Could you check a few things on this drawing? It's one solid part, dimensions in mm from its lowest x, y, z. A direction names the side the tool comes from. Give positions to 0.01 mm unless a question says otherwise; leave off trailing zeros. Order: outer loops, then holes, each group sorted by start corner. A loop starts at its lowest first (then second) coordinate and runs counter-clockwise, first axis right, second up. Notation, with made-up numbers: M 73,24.25 L 115,24.25 A13 cw 115,30.25 Z; hole C 30,53 d9. An arc over 180 degrees is marked long. Return JSON: item names as keys, results as strings. Group by question number.
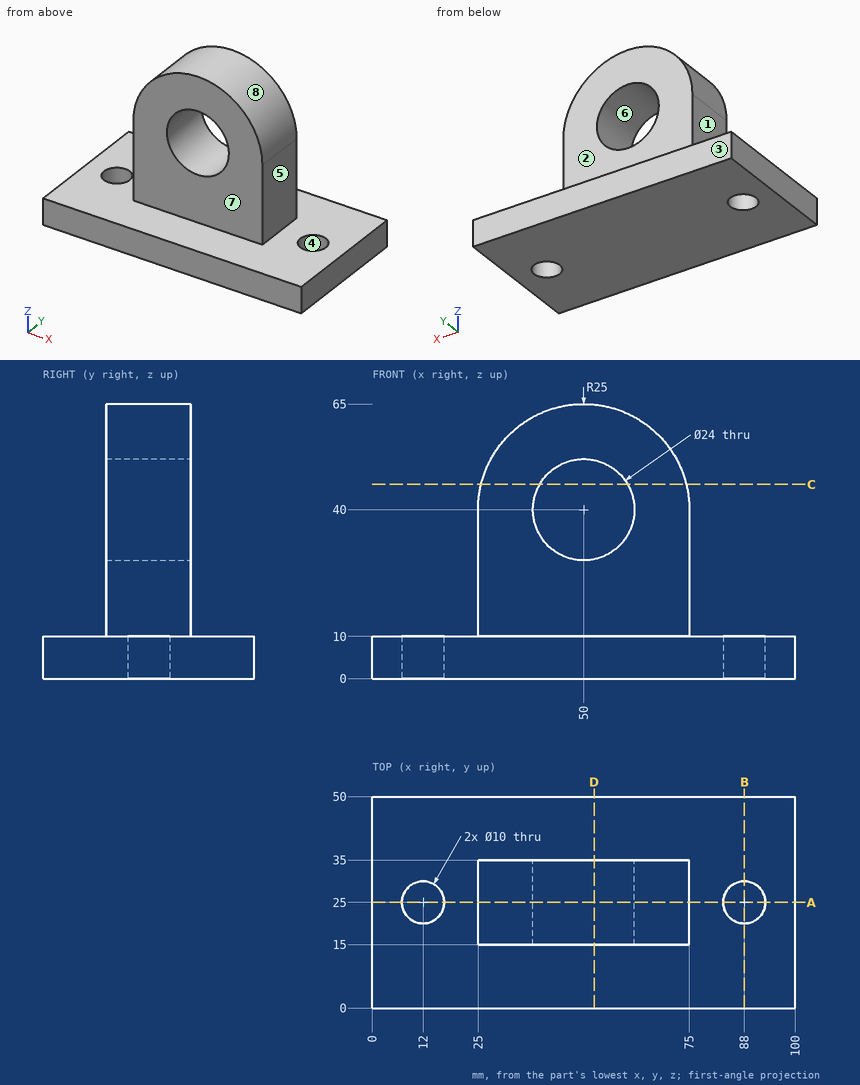
1. Imagine slicing it at A-A, the plane y = 25. Please give me the cut outline in (x, z), plus the area to 3 significant figures.
2. Imagine slicing it at D-D, the plane x = 52.5. Please give me the cut outline in (y, z).
3. Which directions (+Z, -Z, +X, -X, +Y, -Y) give clear straight access to the entire face, cutting with the end or side of a thin tool? Please do the marked faces 1, 2, 3, 4 and 5.
4. Imagine slicing it at C-C, the plane z = 46. Please give me the cut outline in (x, y).
5. I need wall thicknesses on L1, parallel to X at y = 25, z = 7.5; L2, parallel to X at y = 27, z = 40; L3, parallel to Y at x = 12, z = 2.75. Which ranges of each line are inside material? Lowest first, please. Write a range as from..to.
6. For pin 1 (6 mm diameter, centred on x = 38.5, y = 37.5, fed in from -Z); pin 2 (12 mm diameter, centred on x = 79.5, z = 19.5, fed in from -Y); pin 3 (6 mm diameter, centred on x = 31.5, z = 58, fed in from +Y); pin 4 (22 mm diameter, centred on y = 29, z = 23.5, fed in from -X), each with a flat end and sliding along its axis, tell me the tip position at first contact or that it passes through.
7. Imagine slicing it at B-B, the plane x = 88. Please give me the cut outline in (y, z).
8. If we mould it in two halves opening along X, with no side actions, what happens to the marked faces 6, 7 and 8? For each: pulls with the +X half, pulls with the -X half, needs draft (parallel to the pull), parting line crosses it, or undercut.
Values:
{
 "1": {"outline": "M 0,0 L 7,0 L 7,10 L 0,10 Z; M 17,0 L 83,0 L 83,10 L 75,10 L 75,40 A25 ccw 25,40 L 25,10 L 17,10 Z; M 93,0 L 100,0 L 100,10 L 93,10 Z; hole C 50,40 d24", "area": "2,830 mm²"},
 "2": {"outline": "M 0,0 L 50,0 L 50,10 L 35,10 L 35,28.26 L 15,28.26 L 15,10 L 0,10 Z; M 15,51.74 L 35,51.74 L 35,64.87 L 15,64.87 Z"},
 "3": {"face 1": "+Z, -X, +Y, -Y", "face 2": "+Z, +X, -X, +Y", "face 3": "+Z, -Z, +X, -X, +Y", "face 4": "+Z, -Z", "face 5": "+Z, +X, +Y, -Y"},
 "4": {"outline": "M 25.73,15 L 39.61,15 L 39.61,35 L 25.73,35 Z; M 60.39,15 L 74.27,15 L 74.27,35 L 60.39,35 Z"},
 "5": {"L1": "x = 0..7, 17..83, 93..100", "L2": "x = 25..38, 62..75", "L3": "y = 0..20, 30..50"},
 "6": {"pin 1": "stops at z = 0", "pin 2": "stops at y = 15", "pin 3": "stops at y = 35", "pin 4": "stops at x = 25"},
 "7": {"outline": "M 0,0 L 20,0 L 20,10 L 0,10 Z; M 30,0 L 50,0 L 50,10 L 30,10 Z"},
 "8": {"face 6": "undercut", "face 7": "needs draft", "face 8": "parting line crosses it"}
}
